Design review of the part built by this model. Coordinates are the model's own, in mm. Face numbers are marked on the shaded views. A direction names the side the tool comes from. Coordinates: 2 decimals unless noted, no trailing zeros. Loops run counter-clockwise (first coordinate to the right, second up) from the corner with the lowest first, then second, coordinate; pieces in that order, holes last. Notation, with made-up numbers: M 87,48.5 L 137,48.5 A24 ccw 137,76.5 Z; hole C -8,75 d10. An arc over 180 degrees is marked long. Answer as a JSON object with one key per item and string values. Group by question number.
1. Machinability: for the marked faces 1 and 2, which of the approach directions +Z, -Z, +X, -X, +Y, -Y give a long, thin tool a straight path to every point of the face, cutting with its end or side? Answer none if there is none.
2. Draft analysis for pull direction Z (two halves, no side actions). For the marked faces 3, 4 and 5, state which applies: +Z half, -Z half, draft (parallel to the pull), parting line (faces both ways), or undercut.
3. Consider section C-C (z = -7). State the section outline as (x, y) points, then the cut area to 3 significant figures.
4. To check wall thickness, follow probe 1 along Z at (x, y) = (-4, 1.85); probe 2 along Z at (x, y) = (-5.25, 4); probe 3 along Z at (x, y) = (-2.25, 0.7). State the ranges of each line that lie inside material, in increasing order.
5. Consider section B-B (x = -4). State the section outline as (y, z) points.
6. Consider section A-A (y = 2.5). State the section outline as (x, z) points.
7. Insertion check: pin 1 (4 mm diameter, centred on x = -3, z = -18.5, fed in from +Y); pin 2 (0.7 mm diameter, centred on x = -1, y = 3, fed in from -Z). Each pin has a flat end and moves straight along its axis. Give the tip position at first contact, or say it passes through.
Autodesk Inventor part; units mm, degrees
ref_plane "YZ Plane" through (0, 0, 0) normal (1, 0, 0) x (0, 1, 0)
ref_plane "XZ Plane" through (0, 0, 0) normal (0, 1, 0) x (-1, 0, 0)
ref_plane "XY Plane" through (0, 0, 0) normal (0, 0, 1) x (1, 0, 0)
sketch "Esquisse7" plane through (0, 0, 0) normal (0, 1, 0) x (-1, 0, 0)
  line L0 (0, 0) -> (8, 0)
  line L1 (8, 0) -> (8, -10)
  line L2 (8, -10) -> (0, -10)
  line L3 (0, -10) -> (0, 0)
  line L4 (4, -10) -> (4, 0) construction
  circle A0 centre (4, -7) radius 1.7
  dimension "d15" = 3.4
  dimension "d16" = 10
  dimension "d17" = 8
  dimension "d24" = 3
extrude "Extrusion5" add sketch "Esquisse7" along normal blind 5
sketch "Esquisse8" plane through (0, 0, -10) normal (0, 0, -1) x (-1, 0, 0)
  line L0 (8, 5) -> (0, 5) construction
  line L1 (4, 5) -> (4, 0) construction
  line L2 (0, 0) -> (8, 0) construction
  circle A0 centre (4, 2.5) radius 2
  dimension "d20" = 4
extrude "Extrusion6" add sketch "Esquisse8" along normal blind 16
fillet "Congé3" radius 1 1 edges at (-2, 2.5, -10)
sketch "Esquisse9" plane through (-4, 2.5, -26) normal (0, 0, -1) x (-1, 0, 0)
  circle A0 centre (0, 0) radius 2
  arc A1 (-1.6583, 2.5) -> (-1.6583, -2.5) centre (0, 0) ccw
  arc A2 (-1.6583, 2.5) -> (-1.6583, -2.5) centre (0, 0) ccw
  line L0 (-4, 2.5) -> (-1.6583, 2.5)
  line L1 (-4, -2.5) -> (-4, 2.5)
  line L2 (-1.6583, -2.5) -> (-4, -2.5)
  point P0 (-4, -2.5)
properties part number "charniere"
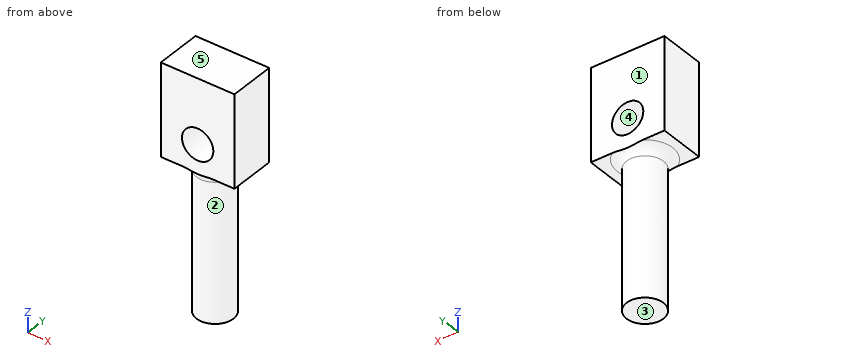
Findings below:
{
 "1": {"face 1": "+Z, -Z, +X, -X, +Y", "face 2": "-Z"},
 "2": {"face 3": "-Z half", "face 4": "undercut", "face 5": "+Z half"},
 "3": {"outline": "M -8,0 L -5.7,0 L -5.7,5 L -8,5 Z; M -2.3,0 L 0,0 L 0,5 L -2.3,5 Z", "area": "23.0 mm^2"},
 "4": {"probe 1": "z = -26 to -8.7, -5.3 to 0", "probe 2": "z = -26 to -8.15, -5.85 to 0", "probe 3": "z = -10.13 to 0"},
 "5": {"outline": "M 0,-10.13 A1 cw 0.5,-11 L 0.5,-26 L 4.5,-26 L 4.5,-11 A1 cw 5,-10.13 L 5,-8.7 L 0,-8.7 Z; M 0,-5.3 L 5,-5.3 L 5,0 L 0,0 Z"},
 "6": {"outline": "M -8,-10 L -7,-10 A1 cw -6,-11 L -6,-26 L -2,-26 L -2,-11 A1 cw -1,-10 L 0,-10 L 0,0 L -8,0 Z; hole C -4,-7 d3.4"},
 "7": {"pin 1": "stops at y = 4.5", "pin 2": "stops at z = -10.05"}
}
